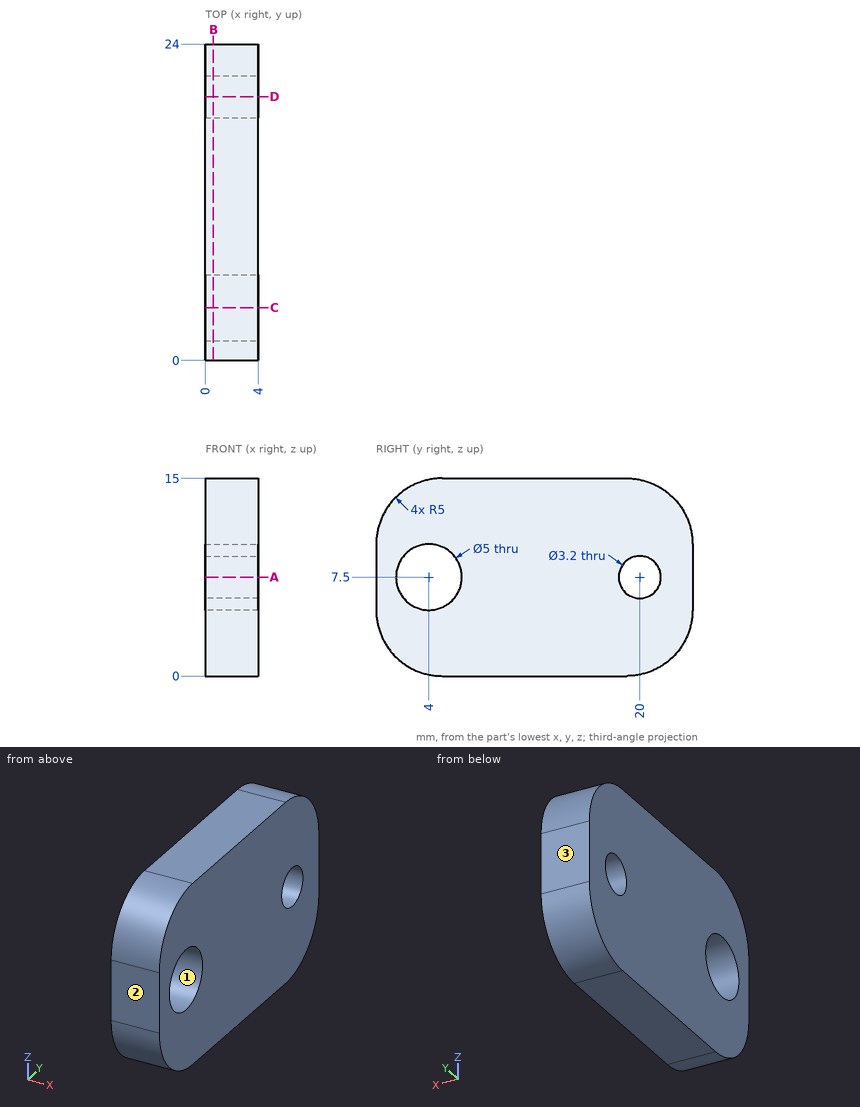
The drawing under review shows one solid part. Ordinate dimensions are in mm from its lowest x, y, z. Give positions to 0.01 mm unless a question says otherwise; leave off trailing zeros. Order: outer loops, then holes, each group sorted by start corner. A loop starts at its lowest first (then second) coordinate and runs counter-clockwise, first axis right, second up. Notation, with made-up numbers: (76, 31.25) - (85, 31.25) arc R20 cw to (85, 66.25) - close; hole circle Ø3 at (-4.5, 9.5). An arc over 180 degrees is marked (long way). Answer as a JSON object with one key per item and string values. Group by question number.
Item 1: Draft analysis for pull direction Y (two halves, no side actions). For the marked faces 1, 2 and 3, state which applies: pulls with the +Y half, pulls with the -Y half, needs draft (parallel to the pull), parting line crosses it, or undercut.
Item 2: Wall thickness on line 1 along Y through (x, z) = (1.75, 7.5); line 2 along Y through (x, z) = (3.15, 7); line 3 along Y through (x, z) = (3.55, 11): over which ranges is each line inside the solid? List them lowest first.
Item 3: Take a section at D-D on y = 20. Give the boundary of the cut face in (x, z).
Item 4: Take a section at A-A on z = 7.5. Give the boundary of the cut face in (x, y), and give its area (3 significant figures).
Item 5: Clearance check with a flat-ended pin moving along its axis: pin 1 Ø1.5 at (x, z) = (3, 3.5) entering from +Y. State where the tip first meets the part, or that it passes through.
Item 6: Take a section at B-B on x = 0.6. Give the boundary of the cut face in (y, z).
Item 7: Take a section at C-C on y = 4. Give the boundary of the cut face in (x, z).
Reported:
{
 "1": {"face 1": "undercut", "face 2": "pulls with the -Y half", "face 3": "pulls with the +Y half"},
 "2": {"line 1": "0 to 1.5, 6.5 to 18.4, 21.6 to 24", "line 2": "0 to 1.55, 6.45 to 18.48, 21.52 to 24", "line 3": "0.1 to 23.9"},
 "3": {"outline": "(0, 0.1) - (4, 0.1) - (4, 5.9) - (0, 5.9) - close; (0, 9.1) - (4, 9.1) - (4, 14.9) - (0, 14.9) - close"},
 "4": {"outline": "(0, 0) - (4, 0) - (4, 1.5) - (0, 1.5) - close; (0, 6.5) - (4, 6.5) - (4, 18.4) - (0, 18.4) - close; (0, 21.6) - (4, 21.6) - (4, 24) - (0, 24) - close", "area": "63.2 mm^2"},
 "5": {"pin 1": "y = 23.94"},
 "6": {"outline": "(0, 5) arc R5 ccw to (5, 0) - (19, 0) arc R5 ccw to (24, 5) - (24, 10) arc R5 ccw to (19, 15) - (5, 15) arc R5 ccw to (0, 10) - close; hole circle Ø5 at (4, 7.5); hole circle Ø3.2 at (20, 7.5)"},
 "7": {"outline": "(0, 0.1) - (4, 0.1) - (4, 5) - (0, 5) - close; (0, 10) - (4, 10) - (4, 14.9) - (0, 14.9) - close"}
}
